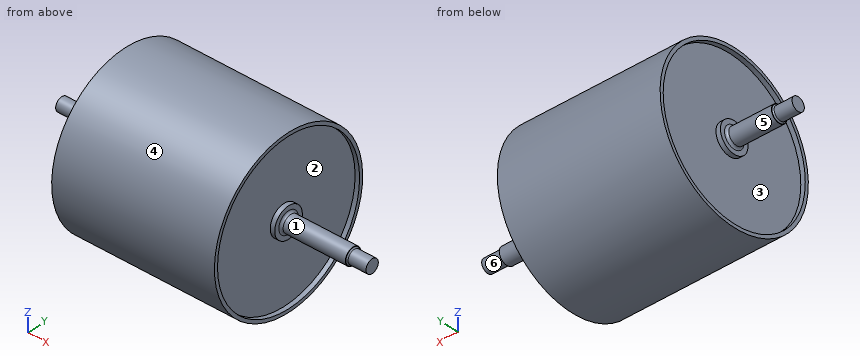
```python
from build123d import *

# Parameters (mm, degrees)
F0_W = 85
F0_H = 30
F2_R = 10
F3_R = 5


with BuildPart() as f1:
    # F0 (on Front) → F1 (revolve)
    with BuildSketch(Plane.XZ):
        with Locations((42.5, 15)):
            Rectangle(F0_W, F0_H)
        Polygon((85, 30), (85, 0), (285, 0), (285, 37.5), (85, 37.5), align=None)
        Polygon((285, 37.5), (285, 0), (465, 0), (465, 50), (355, 50), (285, 50), align=None)
        Polygon((285, 67.5), (285, 50), (355, 50), (355, 67.5), (305, 67.5), align=None)
        Polygon((355, 50), (465, 50), (465, 70), (455, 70), (355, 70), (355, 67.5), align=None)
        Polygon((305, 67.5), (355, 67.5), (355, 70), (355, 170), (355, 347.5), (305, 347.5), align=None)
        Polygon((355, 70), (455, 70), (355, 170), align=None)
        Polygon((285, 347.5), (305, 347.5), (355, 347.5), (647.5, 347.5), (940, 347.5), (990, 347.5), (1010, 347.5), (1010, 362.5), (285, 362.5), align=None)
        Polygon((990, 347.5), (940, 347.5), (940, 170), (940, 70), (940, 67.5), (990, 67.5), align=None)
        Polygon((940, 70), (940, 170), (840, 70), align=None)
        Polygon((1010, 67.5), (990, 67.5), (940, 67.5), (940, 70), (840, 70), (830, 70), (830, 50), (1010, 50), align=None)
        Polygon((1010, 37.5), (1010, 50), (830, 50), (830, 0), (1010, 0), align=None)
        Polygon((1297.5, 37.5), (1010, 37.5), (1010, 0), (1297.5, 0), (1297.5, 30), align=None)
        with Locations((1340, 15)):
            Rectangle(F0_W, F0_H)
    revolve(axis=Axis((691.25, 0, 0), (1, 0, 0)))

    # F2
    f2_edges = [f1.edges().sort_by_distance(p)[0] for p in [
        (1010, 0, -37.5),
        (285, 0, -37.5),
    ]]
    fillet(f2_edges, radius=F2_R)

    # F3
    f3_edges = [f1.edges().sort_by_distance(p)[0] for p in [
        (85, 0, -30),
        (1297.5, 0, -30),
    ]]
    fillet(f3_edges, radius=F3_R)


solid = f1.part
```
Input: part model. Units: mm. Frame: model coordinates. Face numbers are marked on the shaded views. A direction names the side the tool comes from. Give positions to 0.01 mm unless a question says otherwise; leave off trailing zeros. Order: outer loops, then holes, each group sorted by start corner. A loop starts at its lowest first (then second) coordinate and runs counter-clockwise, first axis right, second up. Notation, with made-up numbers: M 48,74 L 73,74 A14 cw 73,88 Z; hole C 24,29 d1. An arc over 180 degrees is marked long. One line per question, with ' | ' between items. Start each with the question number.
1. Material intervals for probe 1 along Y at (x, z) = (300.25, 0); probe 2 along X at (y, z) = (168, 293.5), sorted ascending. Write a range as [from, to].
2. Access query for the marked faces 4, 5 and 6. Directions: +Z, -Z, +X, -X, +Y, -Y. A direction counts if a zero-diameter tool reaches every point of the face in a straight line with its end or side. Return the directions, or none.
3. First-contact query: pin 1 Ø12 at (x, y) = (547, 199) entering from -Z; pin 2 Ø2 at (y, z) = (152.5, -207.5) entering from +X; pin 3 Ø5 at (x, y) = (569, 35) entering from -Z. Flat tips, straight axial feed; report the tip coordinate or a pass-through.
4. Pull-direction query (Z, two-part tool) for the marked faces 1, 2 and 3; classes: released by +Z, released by -Z, zero draft, split by the parting line, or undercut.
5. Section query B-B (z = -242.5). Return the cut outline in (x, y).
6. Section query A-A (y = -284). Return the cut outline in (x, z), and give its area (3 significant figures).
7. Section query C-C (x = 671). Return the cut outline in (y, z).
Here are the results:
1) probe 1: [-362.5, -347.5], [-67.5, 67.5], [347.5, 362.5] | probe 2: [305, 355], [940, 990]
2) face 4: +X, -X | face 5: -X | face 6: +X
3) pin 1: z = -306.85 | pin 2: x = 990 | pin 3: z = -361.04
4) face 1: split by the parting line | face 2: undercut | face 3: undercut
5) outline: M 285,-269.44 L 1010,-269.44 L 1010,-248.9 L 990,-248.9 L 990,248.9 L 1010,248.9 L 1010,269.44 L 285,269.44 L 285,248.9 L 305,248.9 L 305,-248.9 L 285,-248.9 Z; hole M 355,-248.9 L 940,-248.9 L 940,248.9 L 355,248.9 Z
6) outline: M 285,-225.28 L 1010,-225.28 L 1010,-200.25 L 990,-200.25 L 990,200.25 L 1010,200.25 L 1010,225.28 L 285,225.28 L 285,200.25 L 305,200.25 L 305,-200.25 L 285,-200.25 Z; hole M 355,-200.25 L 940,-200.25 L 940,200.25 L 355,200.25 Z | area: 76,300 mm²
7) outline: C 0,0 d725; hole C 0,0 d695
